from build123d import *

# Parameters (mm, degrees)
SKETCH_1_W          = 80
SKETCH_1_H          = 34.45
SKETCH_1_W_2        = 15
SKETCH_1_H_2        = 3
SKETCH_1_W_3        = 30
SKETCH_1_H_3        = 20
SKETCH_1_W_4        = 4
EXTRUDE_1_DEPTH     = 3
SKETCH_2_R          = 2
CUT_EXTRUDE_1_DEPTH = 10
SKETCH_3_W          = 3
SKETCH_3_H          = 4
CUT_EXTRUDE_2_DEPTH = 3


with BuildPart() as part:
    # 草图1 → 凸台-拉伸1 (new body)
    with BuildSketch(Plane(origin=(0, 0, 0), x_dir=(1, 0, 0), z_dir=(0, 1, 0))):
        Rectangle(SKETCH_1_W, SKETCH_1_H)
        with Locations((-17.5, -18.725)):
            Rectangle(SKETCH_1_W_2, SKETCH_1_H_2)
        with Locations((17.5, -18.725)):
            Rectangle(SKETCH_1_W_2, SKETCH_1_H_2)
        with Locations((55, 7.225)):
            Rectangle(SKETCH_1_W_3, SKETCH_1_H_3)
        with Locations((-42, 7.225)):
            Rectangle(SKETCH_1_W_4, SKETCH_1_H_3)
    extrude(amount=EXTRUDE_1_DEPTH)

    # 草图2 → 切除-拉伸1 (cut)
    with BuildSketch(Plane(origin=(0, 3, 0), x_dir=(1, 0, 0), z_dir=(0, 1, 0))):
        with Locations(Location((55.63, 7.225, 0), (0, 0, 270))):
            Circle(SKETCH_2_R)
        with Locations(Location((40.63, 7.225, 0), (0, 0, 270))):
            Circle(SKETCH_2_R)
        with Locations(Location((25.63, 7.225, 0), (0, 0, 270))):
            Circle(SKETCH_2_R)
    extrude(amount=-CUT_EXTRUDE_1_DEPTH, mode=Mode.SUBTRACT)

    # 草图3 → 切除-拉伸2 (cut)
    with BuildSketch(Plane(origin=(0, 3, 0), x_dir=(1, 0, 0), z_dir=(0, 1, 0))):
        with Locations((-38.5, -15.225)):
            Rectangle(SKETCH_3_W, SKETCH_3_H)
        with Locations((38.5, -15.225)):
            Rectangle(SKETCH_3_W, SKETCH_3_H)
    extrude(amount=-CUT_EXTRUDE_2_DEPTH, mode=Mode.SUBTRACT)


solid = part.part
Input: part model. Units: mm. Frame: model coordinates. A direction names the side the tool comes from. Coordinates: 2 decimals unless noted, no trailing zeros. Loops run counter-clockwise (first coordinate to the right, second up) from the corner with the lowest first, then second, coordinate; pieces in that order, holes last. Notation, with made-up numbers: (-26.5, 9.5) -> (8.5, 9.5) arc R28 ccw to (8.5, 32.5) -> close; hole circle Ø1 at (1, 4). An arc over 180 degrees is marked (long way). Write item = value, one per line. Start each with the question number.
Item 1: Mould query, pull axis Z, two halves, no side actions, for faces 6 (the face through (17, 1, 20.225)), 7 (the face through (38.856, 1.521, -6.302)), 8 (the face through (10, 1, 19)), 9 (the face through (23.678, 1.521, -7.659)). Classes: pulls with the +Z half, pulls with the -Z half, needs draft (parallel to the pull), parting line crosses it, or undercut.
Item 2: Cut plane A-A, the plane x = 55.63. Return loops of the section in (y, z) (3 decimals).
Item 3: Material intervals for line 1 (X direction, y = 1.3, z = -7); line 2 (X direction, y = 2.25, z = 5.5); line 3 (X direction, y = 1.35, z = 17), sorted ascending.
Item 4: First-contact query: P1, Ø1.5, axis at y = 1, z = 6.5, coming from the +X side; P2, Ø0.9, axis at y = 1.5, z = 15.5, coming from the +X side; P3, Ø0.9, axis at x = -0.5, y = 1.5, coming from the +Z side (3 decimals). Flat tips, straight axial feed; report the tip coordinate or a pass-through.
Item 5: Cut plane B-B, the plane y = 0.75. Return loops of the section in (x, z) (3 decimals).
Item 6: Reachability of faces 1 (the face through (37, 2, 15)), 2 (the face through (-10, 1, 19)), 3 (the face through (-44, 1, -7)), 4 (the face through (12, 3, -3)), 5 (the face through (-40, 1, 8)) from +Z, -Z, +X, -X, +Y, -Y: full face, straight path, thin tool, end or side. Return the list, or none.
Item 7: Cut plane C-C, the plane x = -32. Return loops of the section in (y, z) (3 decimals), plus the area to 3 significant figures.
Ans:
q1.face_6 = pulls with the +Z half
q1.face_7 = undercut
q1.face_8 = needs draft
q1.face_9 = undercut
q2.outline = (0, -17.225) -> (3, -17.225) -> (3, -9.225) -> (0, -9.225) -> close; (0, -5.225) -> (3, -5.225) -> (3, 2.775) -> (0, 2.775) -> close
q3.line_1 = -44 to 23.64, 27.62 to 38.64, 42.62 to 53.64, 57.62 to 70
q3.line_2 = -40 to 40
q3.line_3 = -37 to 37
q4.P1 = 40
q4.P2 = 37
q4.P3 = 17.225
q5.outline = (-44, -17.225) -> (70, -17.225) -> (70, 2.775) -> (40, 2.775) -> (40, 13.225) -> (37, 13.225) -> (37, 17.225) -> (25, 17.225) -> (25, 20.225) -> (10, 20.225) -> (10, 17.225) -> (-10, 17.225) -> (-10, 20.225) -> (-25, 20.225) -> (-25, 17.225) -> (-37, 17.225) -> (-37, 13.225) -> (-40, 13.225) -> (-40, 2.775) -> (-44, 2.775) -> close; hole circle Ø4 at (25.63, -7.225); hole circle Ø4 at (40.63, -7.225); hole circle Ø4 at (55.63, -7.225)
q6.face_1 = +Z, +X, +Y, -Y
q6.face_2 = +Z, +Y, -Y
q6.face_3 = +Z, -Z, -X, +Y, -Y
q6.face_4 = +Z, -Z, +X, -X, +Y
q6.face_5 = +Z, -X, +Y, -Y
q7.outline = (0, -17.225) -> (3, -17.225) -> (3, 17.225) -> (0, 17.225) -> close
q7.area = 103 mm²
